Part model, mm, in its own coordinate system. A direction names the side the tool comes from. Give positions to 0.01 mm unless a question says otherwise; leave off trailing zeros. Write each loop counter-clockwise with the first axis right and the second up, starting at its lowest first coordinate (ties: lowest second). Pieces come first, ordered by that corner, then holes. Notation, with made-up numbers: M 83.5,-25.75 L 123.5,-25.75 A21 cw 123.5,-18.75 Z; hole C 66,44 d3. An arc over 180 degrees is marked long. Use a Markdown table: item, result.
```python
from build123d import *

# Parameters (mm, degrees)
SKETCH1_W           = 38.1
SKETCH1_H           = 25.4
BOSS_EXTRUDE1_DEPTH = 1.5875
SKETCH3_W           = 9.525
SKETCH3_H           = 25.4
BOSS_EXTRUDE2_DEPTH = 1.5875
SKETCH4_W           = 43.18
SKETCH4_H           = 25.4
BOSS_EXTRUDE3_DEPTH = 1.5875
SKETCH2_R           = 2.0193
CUT_EXTRUDE1_DEPTH  = 2.54
LPATTERN1_COUNT     = 2
LPATTERN1_PITCH     = 25.4


with BuildPart() as part:
    # Sketch1 → Boss-Extrude1 (new body)
    with BuildSketch(Plane.XY):
        with Locations((19.05, 12.7)):
            Rectangle(SKETCH1_W, SKETCH1_H)
    extrude(amount=BOSS_EXTRUDE1_DEPTH)

    # Sketch3 → Boss-Extrude2 (add)
    with BuildSketch(Plane.ZY):
        with Locations((6.35, 12.7)):
            Rectangle(SKETCH3_W, SKETCH3_H)
    extrude(amount=-BOSS_EXTRUDE2_DEPTH)

    # Sketch4 → Boss-Extrude3 (add)
    with BuildSketch(Plane.XY.offset(11.1125)):
        with Locations((-21.59, 12.7)):
            Rectangle(SKETCH4_W, SKETCH4_H)
    extrude(amount=-BOSS_EXTRUDE3_DEPTH)

    # Sketch2 → Cut-Extrude1 (cut)
    with BuildSketch(Plane.XY.offset(1.5875)):
        with Locations((34.29, 12.7)):
            Circle(SKETCH2_R)
    cut_extrude1 = extrude(amount=-CUT_EXTRUDE1_DEPTH, mode=Mode.SUBTRACT)

    # LPattern1: Cut-Extrude1 ×2
    with Locations(*[(-i * LPATTERN1_PITCH, 0, 0) for i in range(1, LPATTERN1_COUNT)]):
        add(cut_extrude1, mode=Mode.SUBTRACT)


solid = part.part
```
1. Drill centre lines: L1, parallel to Y at x = 8.89, z = 0.85; L2, parallel to Z at x = -32.5, y = 7.75 (1 decimal); L3, parallel to Z at x = 7.5, y = 20.5. Where is each one in solid material? Low to high.
Findings below:
| item | result |
|---|---|
| L1 | 0 to 10.68, 14.72 to 25.4 |
| L2 | 9.5 to 11.1 |
| L3 | 0 to 1.59 |
2. Cut at C-C, the plane y = 19.75. Give the cut face in (x, z) (1 decimal).
Findings below:
| item | result |
|---|---|
| outline | M -43.2,9.5 L 0,9.5 L 0,0 L 38.1,0 L 38.1,1.6 L 1.6,1.6 L 1.6,11.1 L -43.2,11.1 Z |
3. Drop flat-ended pins along their axis: P1, Ø12.5, axis at x = -24, y = 19, coming from the -Z side (3 decimals); P2, Ø6, axis at x = 20, z = 7.5, coming from the -Y side; P3, Ø3, axis at y = 11, z = 6.5, coming from the -X side; P4, Ø5, axis at y = 20.5, z = 4.5, coming from the +X side. Give the stop position or say it passes through.
Findings below:
| item | result |
|---|---|
| P1 | z = 9.525 |
| P2 | through |
| P3 | x = 0 |
| P4 | x = 1.59 |
4. Tool access for faces 1 (the flat face through (0, 13, 5)), 2 (the flat face through (0.3, 25.4, 6)), 3 (the flat face through (20, 13, 1.588)): list every direction of +Z, -Z, +X, -X, +Y, -Y with a clear straight run to the whole face (end or side of a thin tool).
Findings below:
| item | result |
|---|---|
| face 1 | -Z, -X, +Y, -Y |
| face 2 | +Z, -Z, +X, -X, +Y |
| face 3 | +Z, +X, +Y, -Y |
5. Cut at D-D, the plane x = -31. Give the cut face in (y, z) (1 decimal).
Findings below:
| item | result |
|---|---|
| outline | M 0,9.5 L 25.4,9.5 L 25.4,11.1 L 0,11.1 Z |
6. Cut at A-A, the plane x = 8.89. Give the cut face in (y, z), then the cut area to 3 significant figures.
Findings below:
| item | result |
|---|---|
| outline | M 0,0 L 10.68,0 L 10.68,1.59 L 0,1.59 Z; M 14.72,0 L 25.4,0 L 25.4,1.59 L 14.72,1.59 Z |
| area | 33.9 mm2 |
7. Cut at B-B, the plane y = 12.7. Give the cut face in (x, z) (1 decimal).
Findings below:
| item | result |
|---|---|
| outline | M -43.2,9.5 L 0,9.5 L 0,0 L 6.9,0 L 6.9,1.6 L 1.6,1.6 L 1.6,11.1 L -43.2,11.1 Z; M 10.9,0 L 32.3,0 L 32.3,1.6 L 10.9,1.6 Z; M 36.3,0 L 38.1,0 L 38.1,1.6 L 36.3,1.6 Z |
8. Two-plate mould, pull along Y, no slides. Class faces 4 (the flat face through (38.1, 13, 1)), 5 (the cylindrical face through (10.755, 11.927, 0.805)), 6 (the flat face through (0.3, 0, 6)), 7 (the cylindrical face through (36.155, 11.927, 0.805)): released by +Y, released by -Y, zero draft, split by the parting line, or undercut.
Findings below:
| item | result |
|---|---|
| face 4 | zero draft |
| face 5 | undercut |
| face 6 | released by -Y |
| face 7 | undercut |
